Design review of the part built by this model. Coordinates are the model's own, in mm. A direction names the side the tool comes from. Coordinates: 2 decimals unless noted, no trailing zeros. Loops run counter-clockwise (first coordinate to the right, second up) from the corner with the lowest first, then second, coordinate; pieces in that order, holes last.
Q1. Draft analysis for pull direction X (two halves, no side actions). For faces 1 (the face through (720, -15, 10)), 2 (the face through (820, -15, 10)), 3 (the face through (463, 0, 172)), 4 (the face through (940, -15, 168)), state which applies: released by +X, released by -X, zero draft, split by the parting line, or undercut.
Q2. Add section A-A on z = 250. Give the boundary of the cut face in (x, y).
Q3. For P1, Ø5.5, axis at x = 470, y = -15, coming from the +Z side; P2, Ø1.8, axis at x = 740.5, z = 225.5, coming from the -Y side; P3, Ø5.5, axis at y = -15, z = 65, coming from the -X side, all flat-tipped, find the tip position at first contact; note any pin that passes through.
Q4. Wall thickness on probe 1 along Z at (x, y) = (937.75, -15); probe 2 along Y at (x, z) = (5, 275); probe 3 along X at (y, z) = (-12.5, 17): over which ranges is each line inside the solid? List them lowest first.
Q5. Machinability: for faces 5 (the face through (171, -15, 20)), 6 (the face through (463, -30, 172)), which of the approach directions +Z, -Z, +X, -X, +Y, -Y give a long, thin tool a straight path to every point of the face, cutting with its end or side? Answer none if there is none.
```python
from build123d import *

# Parameters (mm, degrees)
F0_W      = 940
F0_H      = 340
F1_DEPTH  = 30
F2_R      = 3
F3_DEPTH  = 12
F4_W      = 100
F4_H      = 20
F5_DEPTH  = 30
F6_W      = 100
F6_H      = 20
F7_DEPTH  = 30
F8_R      = 35
F9_DEPTH  = 30
F11_R     = 3
F12_DEPTH = 12
F13_R     = 3
F14_DEPTH = 12
F15_R     = 3
F16_DEPTH = 12


with BuildPart() as f1:
    # F0 (on Front) → F1 (new body)
    with BuildSketch(Plane.XZ):
        with Locations((470, 170)):
            Rectangle(F0_W, F0_H)
    extrude(amount=F1_DEPTH)

    # F2 (on face) → F3 (cut)
    with BuildSketch(Plane.XY.offset(340)):
        with Locations((470, -15)):
            Circle(F2_R)
    extrude(amount=-F3_DEPTH, mode=Mode.SUBTRACT)

    # F4 (on face) → F5 (cut)
    with BuildSketch(Plane(origin=(0, 0, 0), x_dir=(-1, 0, 0), z_dir=(0, 1, 0))):
        with Locations((-770, 10)):
            Rectangle(F4_W, F4_H)
    extrude(amount=-F5_DEPTH, mode=Mode.SUBTRACT)

    # F6 (on face) → F7 (cut)
    with BuildSketch(Plane(origin=(0, 0, 0), x_dir=(-1, 0, 0), z_dir=(0, 1, 0))):
        with Locations((-170, 10)):
            Rectangle(F6_W, F6_H)
    extrude(amount=-F7_DEPTH, mode=Mode.SUBTRACT)

    # F8 (on face) → F9 (cut)
    with BuildSketch(Plane(origin=(0, 0, 0), x_dir=(-1, 0, 0), z_dir=(0, 1, 0))):
        with Locations((-470, 250)):
            Circle(F8_R)
    extrude(amount=-F9_DEPTH, mode=Mode.SUBTRACT)

    # F11 (on face) → F12 (cut)
    with BuildSketch(Plane.YZ.offset(940)):
        with Locations((-15, 275)):
            Circle(F11_R)
        with Locations((-15, 65)):
            Circle(F11_R)
    extrude(amount=-F12_DEPTH, mode=Mode.SUBTRACT)

    # F13 (on face) → F14 (cut)
    with BuildSketch(Plane(origin=(0, 0, 0), x_dir=(0, -1, 0), z_dir=(-1, 0, 0))):
        with Locations((15, 275)):
            Circle(F13_R)
        with Locations((15, 65)):
            Circle(F13_R)
    extrude(amount=-F14_DEPTH, mode=Mode.SUBTRACT)

    # F15 (on face) → F16 (cut)
    with BuildSketch(Plane.XZ.offset(30)):
        with Locations((740, 225)):
            Circle(F15_R)
        with Locations((200, 225)):
            Circle(F15_R)
    extrude(amount=-F16_DEPTH, mode=Mode.SUBTRACT)


solid = f1.part
```
Entries:
1. face 1: undercut
1. face 2: undercut
1. face 3: zero draft
1. face 4: released by +X
2. outline: (0, -30) - (435, -30) - (435, 0) - (0, 0) - close; (505, -30) - (940, -30) - (940, 0) - (505, 0) - close
3. P1: stops at z = 328
3. P2: stops at y = -18
3. P3: stops at x = 12
4. probe 1: z = 0 to 62, 68 to 272, 278 to 340
4. probe 2: y = -30 to -18, -12 to 0
4. probe 3: x = 0 to 120, 220 to 720, 820 to 940
5. face 5: -Z, +Y, -Y
5. face 6: +Z, -Z, +X, -X, -Y
